Verification items for the finished model (mm, model axes). A direction names the side the tool comes from. Round coordinates to 2 decimals unless told otherwise and drop trailing zeros. Write each loop counter-clockwise with the first axis right and the second up, starting at its lowest first coordinate (ties: lowest second). Pieces come first, ordered by that corner, then holes.
from build123d import *

# Parameters (mm, degrees)
SKETCH_1_W          = 63.76
SKETCH_1_H          = 52.92
EXTRUDE_1_DEPTH     = 1
FILLET_1_R          = 1
SKETCH_2_W          = 25.4
SKETCH_2_H          = 5.54
EXTRUDE_2_DEPTH     = 0.5
CHAMFER_1_SIZE      = 0.5
SKETCH_3_R          = 0.8
CUT_EXTRUDE_2_DEPTH = 52.633662839
EXTRUDE_START       = 3
SKETCH_4_W          = 61.76
SKETCH_4_H          = 50.92
EXTRUDE_3_DEPTH     = 3


with BuildPart() as part:
    # 草图1 → 凸台-拉伸1 (new body)
    with BuildSketch(Plane(origin=(0, 0, 0), x_dir=(1, 0, 0), z_dir=(0, 1, 0))):
        with Locations((-7.873913043, -6.455217391)):
            Rectangle(SKETCH_1_W, SKETCH_1_H)
    extrude(amount=EXTRUDE_1_DEPTH)

    # 圆角1
    fillet_1_edges = [part.edges().sort_by_distance(p)[0] for p in [
        (-39.753913043, 0.5, -20.004782609),
        (24.006086957, 0.5, -20.004782609),
        (24.006086957, 0.5, 32.915217391),
        (-39.753913043, 0.5, 32.915217391),
    ]]
    fillet(fillet_1_edges, radius=FILLET_1_R)

    # 草图2 → 凸台-拉伸2 (add)
    with BuildSketch(Plane(origin=(0, 1, 0), x_dir=(1, 0, 0), z_dir=(0, 1, 0))):
        with Locations((-7.924409429, 10.034782609)):
            Rectangle(SKETCH_2_W, SKETCH_2_H)
        with Locations((-7.883913043, -16.965217391)):
            Rectangle(SKETCH_2_W, SKETCH_2_H)
    extrude(amount=EXTRUDE_2_DEPTH)

    # 倒角1
    chamfer_1_edges = [part.edges().sort_by_distance(p)[0] for p in [
        (4.816086957, 1, 16.965217391),
        (-7.883913043, 1, 14.195217391),
        (-7.883913043, 1, 19.735217391),
        (-20.583913043, 1, 16.965217391),
        (-20.624409429, 1, -10.034782609),
        (-7.924409429, 1, -12.804782609),
        (4.775590571, 1, -10.034782609),
        (-7.924409429, 1, -7.264782609),
    ]]
    chamfer(chamfer_1_edges, length=CHAMFER_1_SIZE - 0.0001)  # a hair under: the kernel refuses the full size

    # 草图3 → 切除-拉伸2 (cut, through all)
    with BuildSketch(Plane.XZ):
        with Locations(Location((-19.313913043, 18.465217391, 0), (0, 0, 270))):
            Circle(SKETCH_3_R)
        with Locations(Location((-16.773913043, 18.465217391, 0), (0, 0, 270))):
            Circle(SKETCH_3_R)
        with Locations(Location((-14.233913043, 18.465217391, 0), (0, 0, 270))):
            Circle(SKETCH_3_R)
        with Locations(Location((-11.693913043, 18.465217391, 0), (0, 0, 270))):
            Circle(SKETCH_3_R)
        with Locations(Location((-9.153913043, 18.465217391, 0), (0, 0, 270))):
            Circle(SKETCH_3_R)
        with Locations(Location((-6.613913043, 18.465217391, 0), (0, 0, 270))):
            Circle(SKETCH_3_R)
        with Locations(Location((-4.073913043, 18.465217391, 0), (0, 0, 270))):
            Circle(SKETCH_3_R)
        with Locations(Location((-1.533913043, 18.465217391, 0), (0, 0, 270))):
            Circle(SKETCH_3_R)
        with Locations(Location((1.006086957, 18.465217391, 0), (0, 0, 270))):
            Circle(SKETCH_3_R)
        with Locations(Location((3.546086957, 18.465217391, 0), (0, 0, 270))):
            Circle(SKETCH_3_R)
        with Locations(Location((-16.773913043, 15.465217391, 0), (0, 0, 270))):
            Circle(SKETCH_3_R)
        with Locations(Location((-14.233913043, 15.465217391, 0), (0, 0, 270))):
            Circle(SKETCH_3_R)
        with Locations(Location((-11.693913043, 15.465217391, 0), (0, 0, 270))):
            Circle(SKETCH_3_R)
        with Locations(Location((-9.153913043, 15.465217391, 0), (0, 0, 270))):
            Circle(SKETCH_3_R)
        with Locations(Location((-6.613913043, 15.465217391, 0), (0, 0, 270))):
            Circle(SKETCH_3_R)
        with Locations(Location((-4.073913043, 15.465217391, 0), (0, 0, 270))):
            Circle(SKETCH_3_R)
        with Locations(Location((-1.533913043, 15.465217391, 0), (0, 0, 270))):
            Circle(SKETCH_3_R)
        with Locations(Location((1.006086957, 15.465217391, 0), (0, 0, 270))):
            Circle(SKETCH_3_R)
        with Locations(Location((3.546086957, 15.465217391, 0), (0, 0, 270))):
            Circle(SKETCH_3_R)
        with Locations(Location((-19.313913043, 15.465217391, 0), (0, 0, 270))):
            Circle(SKETCH_3_R)
        with Locations(Location((-19.313913043, -8.534782609, 0), (0, 0, 270))):
            Circle(SKETCH_3_R)
        with Locations(Location((-16.773913043, -8.534782609, 0), (0, 0, 270))):
            Circle(SKETCH_3_R)
        with Locations(Location((-14.233913043, -8.534782609, 0), (0, 0, 270))):
            Circle(SKETCH_3_R)
        with Locations(Location((-11.693913043, -8.534782609, 0), (0, 0, 270))):
            Circle(SKETCH_3_R)
        with Locations(Location((-9.153913043, -8.534782609, 0), (0, 0, 270))):
            Circle(SKETCH_3_R)
        with Locations(Location((-6.613913043, -8.534782609, 0), (0, 0, 270))):
            Circle(SKETCH_3_R)
        with Locations(Location((-4.073913043, -8.534782609, 0), (0, 0, 270))):
            Circle(SKETCH_3_R)
        with Locations(Location((-1.533913043, -8.534782609, 0), (0, 0, 270))):
            Circle(SKETCH_3_R)
        with Locations(Location((1.006086957, -8.534782609, 0), (0, 0, 270))):
            Circle(SKETCH_3_R)
        with Locations(Location((3.546086957, -8.534782609, 0), (0, 0, 270))):
            Circle(SKETCH_3_R)
        with Locations(Location((-16.773913043, -11.534782609, 0), (0, 0, 270))):
            Circle(SKETCH_3_R)
        with Locations(Location((-14.233913043, -11.534782609, 0), (0, 0, 270))):
            Circle(SKETCH_3_R)
        with Locations(Location((-11.693913043, -11.534782609, 0), (0, 0, 270))):
            Circle(SKETCH_3_R)
        with Locations(Location((-9.153913043, -11.534782609, 0), (0, 0, 270))):
            Circle(SKETCH_3_R)
        with Locations(Location((-6.613913043, -11.534782609, 0), (0, 0, 270))):
            Circle(SKETCH_3_R)
        with Locations(Location((-4.073913043, -11.534782609, 0), (0, 0, 270))):
            Circle(SKETCH_3_R)
        with Locations(Location((-1.533913043, -11.534782609, 0), (0, 0, 270))):
            Circle(SKETCH_3_R)
        with Locations(Location((1.006086957, -11.534782609, 0), (0, 0, 270))):
            Circle(SKETCH_3_R)
        with Locations(Location((3.546086957, -11.534782609, 0), (0, 0, 270))):
            Circle(SKETCH_3_R)
        with Locations(Location((-19.313913043, -11.534782609, 0), (0, 0, 270))):
            Circle(SKETCH_3_R)
    extrude(amount=-CUT_EXTRUDE_2_DEPTH, mode=Mode.SUBTRACT)

    # 草图4 → 凸台-拉伸3 (add)
    with BuildSketch(Plane(origin=(0, 1, 0), x_dir=(1, 0, 0), z_dir=(0, 1, 0)).offset(EXTRUDE_START)):
        with BuildLine():
            Line((-38.753913043, -32.915217391), (23.006086957, -32.915217391))
            ThreePointArc((23.006086957, -32.915217391), (23.713193738, -32.622324172), (24.006086957, -31.915217391))
            Line((24.006086957, -31.915217391), (24.006086957, 19.004782609))
            ThreePointArc((24.006086957, 19.004782609), (23.713193738, 19.71188939), (23.006086957, 20.004782609))
            Line((23.006086957, 20.004782609), (-38.753913043, 20.004782609))
            ThreePointArc((-38.753913043, 20.004782609), (-39.461019825, 19.71188939), (-39.753913043, 19.004782609))
            Line((-39.753913043, 19.004782609), (-39.753913043, -31.915217391))
            ThreePointArc((-39.753913043, -31.915217391), (-39.461019825, -32.622324172), (-38.753913043, -32.915217391))
        make_face()
        with Locations((-7.873913043, -6.455217391)):
            Rectangle(SKETCH_4_W, SKETCH_4_H, mode=Mode.SUBTRACT)
    extrude(amount=-EXTRUDE_3_DEPTH)


solid = part.part
Q1. Sectioned sample at C-C (z = 1.5). Enter the section's corners in (x, y).
Recorded:
outline: (-39.75, 0) - (24.01, 0) - (24.01, 4) - (23.01, 4) - (23.01, 1) - (-38.75, 1) - (-38.75, 4) - (-39.75, 4) - close
Q2. Release check for a two-part mould opening along Z. For faces 3 (the flat face through (-8, 0, 6)), 4 (the cylindrical face through (-16.739, 0.74, -7.736)) record: released by +Z, released by -Z, zero draft, split by the parting line, or undercut.
Recorded:
face 3: zero draft
face 4: undercut
Q3. Material ranges on line 1 along Z through (x, y) = (11.5, 1.85); line 2 along X through (y, z) = (2.75, -16); line 3 along Y through (x, z) = (-9.5, 0.5), recorded low to high.
Recorded:
line 1: z = -20 to -19, 31.92 to 32.92
line 2: x = -39.75 to -38.75, 23.01 to 24.01
line 3: y = 0 to 1
Q4. Depth check by flat-ended pin: P1, Ø1, axis at x = -9.15, z = -11.53, coming from the -Y side; P2, Ø2.5, axis at x = -6.61, z = 15.47, coming from the +Y side. Enter the tip coordinate at first touch or a pass-through.
Recorded:
P1: passes through
P2: stops at y = 1.5
Q5. Sectioned sample at B-B (x = 11). Enter the section's corners in (y, z), plus the area to 3 significant figures.
Recorded:
outline: (0, -20) - (4, -20) - (4, -19) - (1, -19) - (1, 31.92) - (4, 31.92) - (4, 32.92) - (0, 32.92) - close
area: 58.9 mm2
Q6. Sectioned sample at A-A (y = 3.1). Enter the section's corners in (x, z).
Recorded:
outline: (-39.75, -19) arc R1 ccw to (-38.75, -20) - (23.01, -20) arc R1 ccw to (24.01, -19) - (24.01, 31.92) arc R1 ccw to (23.01, 32.92) - (-38.75, 32.92) arc R1 ccw to (-39.75, 31.92) - close; hole (-38.75, -19) - (23.01, -19) - (23.01, 31.92) - (-38.75, 31.92) - close
Q7. Tool access check on faces 1 (the flat face through (-8, 1, 6)), 2 (the cylindrical face through (3.06, 0.74, -7.9)). Record the directions out of +Z, -Z, +X, -X, +Y, -Y that give a thin tool (end or side, any length) a straight path to the whole face; none if there is none.
Recorded:
face 1: +Y
face 2: +Y, -Y
